```python
from build123d import *

# Parameters (mm, degrees)
BOSS_EXTRUDE1_DEPTH = 5
SKETCH2_R           = 6
CUT_EXTRUDE1_DEPTH  = 96.818839484
SKETCH3_R           = 8
CUT_EXTRUDE2_DEPTH  = 4
SKETCH4_R           = 1.75
CUT_EXTRUDE3_DEPTH  = 96.818839484
CUT_EXTRUDE4_DEPTH  = 2
SKETCH6_R           = 1.75
CUT_EXTRUDE5_DEPTH  = 96.818839484


with BuildPart() as part:
    # Sketch1 → Boss-Extrude1 (new body)
    with BuildSketch(Plane.XY):
        with BuildLine():
            Line((-32.5, 0), (-32.5, 90))
            Line((-32.5, 90), (32.5, 90))
            Line((32.5, 90), (32.5, 0))
            ThreePointArc((32.5, 0), (0, -32.5), (-32.5, 0))
        make_face()
    extrude(amount=BOSS_EXTRUDE1_DEPTH)

    # Sketch2 → Cut-Extrude1 (cut, through all)
    with BuildSketch(Plane.XY.offset(5)):
        Circle(SKETCH2_R)
    extrude(amount=-CUT_EXTRUDE1_DEPTH, mode=Mode.SUBTRACT)

    # Sketch3 → Cut-Extrude2 (cut)
    with BuildSketch(Plane.XY.offset(5)):
        Circle(SKETCH3_R)
    extrude(amount=-CUT_EXTRUDE2_DEPTH, mode=Mode.SUBTRACT)

    # Sketch4 → Cut-Extrude3 (cut, through all)
    with BuildSketch(Plane.XY.offset(5)):
        with Locations((-12, 12)):
            Circle(SKETCH4_R)
        with Locations(Location((12, 12, 0), (0, 0, 180))):
            Circle(SKETCH4_R)
        with Locations((12, -12)):
            Circle(SKETCH4_R)
        with Locations(Location((-12, -12, 0), (0, 0, 180))):
            Circle(SKETCH4_R)
    extrude(amount=-CUT_EXTRUDE3_DEPTH, mode=Mode.SUBTRACT)

    # Sketch5 → Cut-Extrude4 (cut)
    with BuildSketch(Plane.XY.offset(5)):
        Polygon((-8.709103466, 12), (-10.354551733, 14.85), (-13.645448267, 14.85), (-15.290896534, 12), (-13.645448267, 9.15), (-10.354551733, 9.15), align=None)
        Polygon((10.354551733, 9.15), (8.709103466, 12), (10.354551733, 14.85), (13.645448267, 14.85), (15.290896534, 12), (13.645448267, 9.15), align=None)
        Polygon((8.709103466, -12), (10.354551733, -14.85), (13.645448267, -14.85), (15.290896534, -12), (13.645448267, -9.15), (10.354551733, -9.15), align=None)
        Polygon((-10.354551733, -9.15), (-8.709103466, -12), (-10.354551733, -14.85), (-13.645448267, -14.85), (-15.290896534, -12), (-13.645448267, -9.15), align=None)
    extrude(amount=-CUT_EXTRUDE4_DEPTH, mode=Mode.SUBTRACT)

    # Sketch6 → Cut-Extrude5 (cut, through all)
    with BuildSketch(Plane.XY.offset(5)):
        with Locations((-27.5, 62.5)):
            Circle(SKETCH6_R)
        with Locations((-27.5, 54)):
            Circle(SKETCH6_R)
        with Locations(Location((27.5, 54, 0), (0, 0, 180))):
            Circle(SKETCH6_R)
        with Locations(Location((27.5, 62.5, 0), (0, 0, 180))):
            Circle(SKETCH6_R)
    extrude(amount=-CUT_EXTRUDE5_DEPTH, mode=Mode.SUBTRACT)


solid = part.part
```
The listing builds one solid part. Answer for the finished solid, in the listing's coordinates (mm). A direction names the side the tool comes from. Round coordinates to 2 decimals unless told otherwise and drop trailing zeros. Loops run counter-clockwise (first coordinate to the right, second up) from the corner with the lowest first, then second, coordinate; pieces in that order, holes last. Notation, with made-up numbers: (82.5, 33) -> (120.5, 33) arc R16 cw to (120.5, 46) -> close; hole circle Ø6 at (9, -14.5). An arc over 180 degrees is marked (long way). Use one line per item in the form item = value.
1. The part is cut by section D-D on x = 12. Determine the outline of the cut face in (y, z), and give its area (3 significant figures).
Answer key:
outline = (-30.2, 0) -> (-13.75, 0) -> (-13.75, 3) -> (-14.85, 3) -> (-14.85, 5) -> (-30.2, 5) -> close; (-10.25, 0) -> (10.25, 0) -> (10.25, 3) -> (9.15, 3) -> (9.15, 5) -> (-9.15, 5) -> (-9.15, 3) -> (-10.25, 3) -> close; (13.75, 0) -> (90, 0) -> (90, 5) -> (14.85, 5) -> (14.85, 3) -> (13.75, 3) -> close
area = 557 mm²
2. Flat-ended cylindrical pins translate along their axes: pin 1 Ø1.7 at (x, y) = (13.5, 11) entering from +Z; pin 2 Ø2 at (x, z) = (12, 3.5) entering from -Y; pin 3 Ø1 at (x, z) = (-12.5, 3.5) entering from -Y; pin 4 Ø3 at (x, y) = (12, 12) entering from +Z. Find the tip coordinate at first contact, or state that the pin passes through.
Answer key:
pin_1 = 3
pin_2 = -30.58
pin_3 = -30.2
pin_4 = through
3. The part is cut by section A-A on x = 0. Determine the outline of the cut face in (y, z).
Answer key:
outline = (-32.5, 0) -> (-6, 0) -> (-6, 1) -> (-8, 1) -> (-8, 5) -> (-32.5, 5) -> close; (6, 0) -> (90, 0) -> (90, 5) -> (8, 5) -> (8, 1) -> (6, 1) -> close
4. The part is cut by section C-C on x = -27.5. Determine the outline of the cut face in (y, z), and give its area (3 significant figures).
Answer key:
outline = (-17.32, 0) -> (52.25, 0) -> (52.25, 5) -> (-17.32, 5) -> close; (55.75, 0) -> (60.75, 0) -> (60.75, 5) -> (55.75, 5) -> close; (64.25, 0) -> (90, 0) -> (90, 5) -> (64.25, 5) -> close
area = 502 mm²
5. Find the intervals of material crossed by probe 1 along Y at (x, z) = (-28, 3.6); probe 2 along Y at (x, z) = (-27.5, 0.45); probe 3 along Z at (x, y) = (-6.5, -0.5), in increasing order. Write a range as [from, to].
Answer key:
probe_1 = [-16.5, 52.32], [55.68, 60.82], [64.18, 90]
probe_2 = [-17.32, 52.25], [55.75, 60.75], [64.25, 90]
probe_3 = [0, 1]
6. The part is cut by section B-B on z = 4.05. Give the number of separate pieces and of enclosed holes in the cut face, and give its area (3 significant figures).
Answer key:
separate_pieces = 1
enclosed_holes = 9
area = 7,160 mm²
7. A tool of negligible diameter and unlimited length cuts with its end or side. For faces 4 (the cylindrical face through (-5.994, 0.264, 0.507)), 5 (the flat face through (13.4, -10.7, 3)), from which of +Z, -Z, +X, -X, +Y, -Y can it reach the whole face along a straight path? Write none if from no direction.
Answer key:
face_4 = +Z, -Z
face_5 = +Z
8. For a pull along Y with two mould halves and no side action, classify faces 1 (the flat face through (32.5, 46, 2)), 2 (the cylindrical face through (12.9, -10.5, 1.5)), 3 (the flat face through (0, 90, 2)) as released by +Y, released by -Y, zero draft, split by the parting line, or undercut.
Answer key:
face_1 = zero draft
face_2 = undercut
face_3 = released by +Y
